Geometry check sheet. Reference: drawing and pictorial views, mm from the part's lowest x, y, z. Give positions to 0.01 mm unless a question says otherwise; leave off trailing zeros. Loops run counter-clockwise (first coordinate to the right, second up) from the corner with the lowest first, then second, coordinate; pieces in that order, holes last. Notation, with made-up numbers: (83.5, -10.75) - (118.5, -10.75) arc R34 ccw to (118.5, 23.25) - close; hole circle Ø1 at (46, 23). An arc over 180 degrees is marked (long way). Answer in a Markdown table with one row per item. Add a question column.
(1) Draft check along Y on the marked faces 1, 2, 3 and 4. Enter one of: released by +Y, released by -Y, zero draft, split by the parting line, or undercut.
(2) Go/stop test with flat-tipped pins: P1, Ø5, axis at x = 189.5, y = 341, coming from the +Z side; P2, Ø12.5, axis at y = 241.5, z = 117.5, coming from the +X side; P3, Ø10, axis at y = 279, z = 208.5, coming from the +X side. Record where each tip stops, or that it passes through.
(3) Sectioned sample at D-D on z = 186.5. Enter the section's corners in (x, y) (1 decimal), then the cut area to 3 significant figures.
(4) Sectioned sample at A-A on z = 138. Enter the section's corners in (x, y) (1 decimal), then the cut area to 3 significant figures.
(5) Thickness scan on L1, parallel to Y at x = 232.5, z = 133 (1 decimal); L2, parallel to Y at x = 171, z = 164 (1 decimal); L3, parallel to Z at x = 191, y = 242. Record the ranges inside material, lowest first.
(6) Sectioned sample at B-B on y = 37.5. Enter the section's corners in (x, z) (1 decimal).
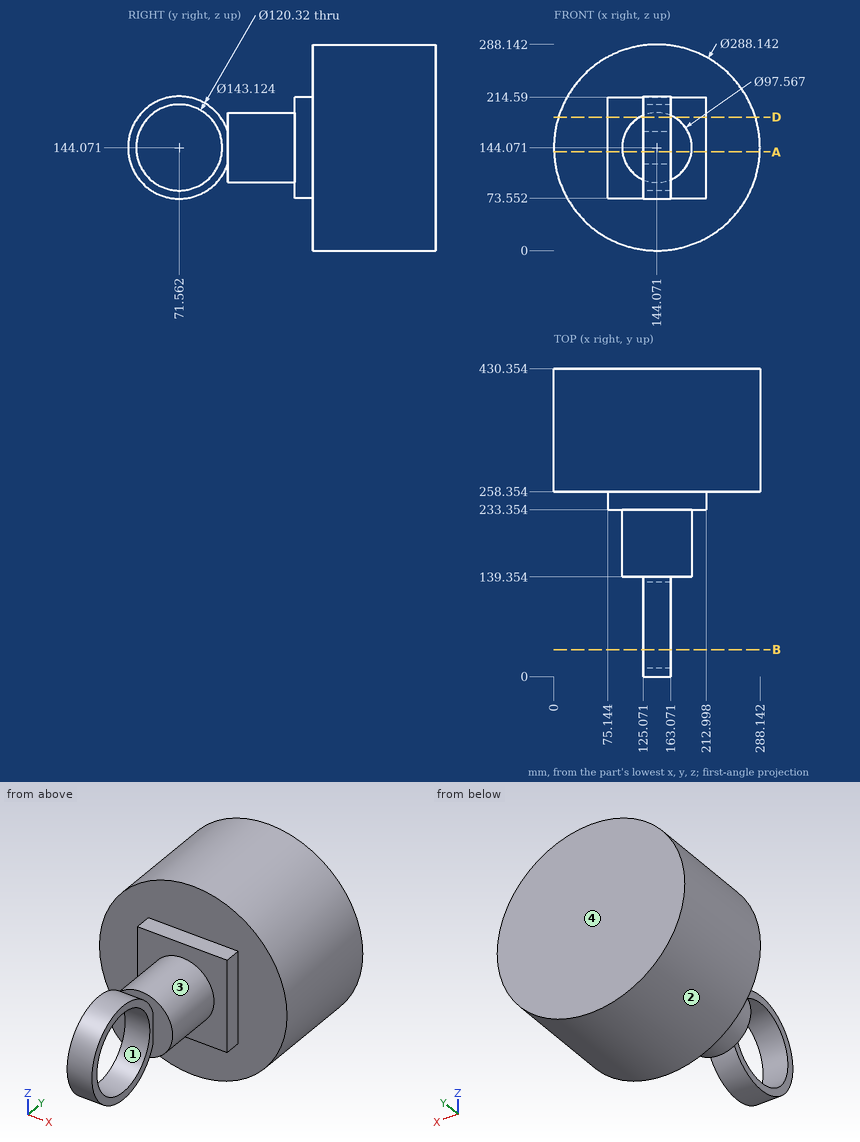
Reply:
| question | item | result |
|---|---|---|
| 1 | face 1 | undercut |
| 1 | face 2 | zero draft |
| 1 | face 3 | undercut |
| 1 | face 4 | released by +Y |
| 2 | P1 | z = 281.6 |
| 2 | P2 | x = 213 |
| 2 | P3 | x = 275.31 |
| 3 | outline | (6.4, 258.4) - (75.1, 258.4) - (75.1, 233.4) - (120, 233.4) - (120, 139.4) - (168.1, 139.4) - (168.1, 233.4) - (213, 233.4) - (213, 258.4) - (281.8, 258.4) - (281.8, 430.4) - (6.4, 430.4) - close; (125.1, 13.9) - (163.1, 13.9) - (163.1, 28.9) - (125.1, 28.9) - close; (125.1, 114.2) - (163.1, 114.2) - (163.1, 129.2) - (125.1, 129.2) - close |
| 3 | area | 56,500 mm^2 |
| 4 | outline | (0.1, 258.4) - (75.1, 258.4) - (75.1, 233.4) - (95.7, 233.4) - (95.7, 139.4) - (125.1, 139.4) - (125.1, 131.4) - (163.1, 131.4) - (163.1, 139.4) - (192.5, 139.4) - (192.5, 233.4) - (213, 233.4) - (213, 258.4) - (288, 258.4) - (288, 430.4) - (0.1, 430.4) - close; (125.1, 0.3) - (163.1, 0.3) - (163.1, 11.7) - (125.1, 11.7) - close |
| 4 | area | 62,800 mm^2 |
| 5 | L1 | 258.4 to 430.4 |
| 5 | L2 | 139.4 to 430.4 |
| 5 | L3 | 73.55 to 214.59 |
| 6 | outline | (125.1, 81.1) - (163.1, 81.1) - (163.1, 94.5) - (125.1, 94.5) - close; (125.1, 193.7) - (163.1, 193.7) - (163.1, 207) - (125.1, 207) - close |
